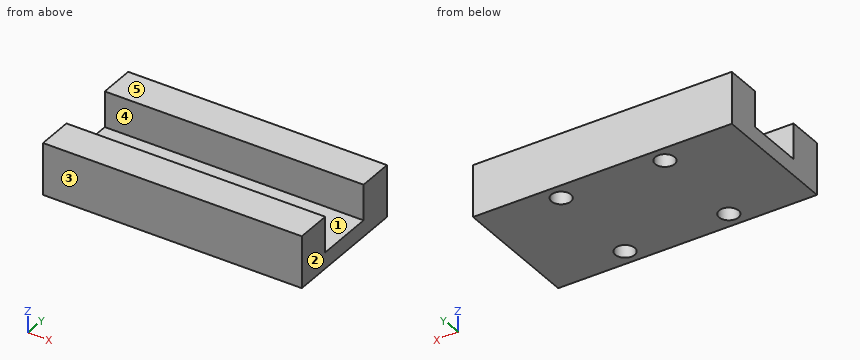
```python
from build123d import *

# Parameters (mm, degrees)
SKETCH_1_W          = 39.9
SKETCH_1_H          = 20
EXTRUDE_1_DEPTH     = 8
SKETCH_2_R          = 1.5
CUT_EXTRUDE_1_DEPTH = 3
SKETCH_3_W          = 5.5
SKETCH_3_H          = 9
CUT_EXTRUDE_2_DEPTH = 46.343246465


with BuildPart() as part:
    # 草图1 → 凸台-拉伸1 (new body)
    with BuildSketch(Plane.XY):
        with Locations((-19.95, 10)):
            Rectangle(SKETCH_1_W, SKETCH_1_H)
    extrude(amount=EXTRUDE_1_DEPTH)

    # 草图2 → 切除-拉伸1 (cut)
    with BuildSketch(Plane(origin=(0, 0, 0), x_dir=(-1, 0, 0), z_dir=(0, 0, -1))):
        with Locations((11.95, 17.5)):
            Circle(SKETCH_2_R)
        with Locations((27.95, 17.5)):
            Circle(SKETCH_2_R)
        with Locations(Location((27.95, 2.5, 0), (0, 0, 180))):
            Circle(SKETCH_2_R)
        with Locations(Location((11.95, 2.5, 0), (0, 0, 180))):
            Circle(SKETCH_2_R)
    extrude(amount=-CUT_EXTRUDE_1_DEPTH, mode=Mode.SUBTRACT)

    # 草图3 → 切除-拉伸2 (cut, through all)
    with BuildSketch(Plane(origin=(0, 0, 0), x_dir=(0, 0, -1), z_dir=(1, 0, 0))):
        with Locations((-5.25, 10)):
            Rectangle(SKETCH_3_W, SKETCH_3_H)
    extrude(amount=-CUT_EXTRUDE_2_DEPTH, mode=Mode.SUBTRACT)


solid = part.part
```
Check sheet for the modelled part. Datum: model origin and axes. Units: mm. Face numbers are marked on the shaded views. A direction names the side the tool comes from. Round coordinates to 2 decimals unless told otherwise and drop trailing zeros. Order: outer loops, then holes, each group sorted by start corner. A loop starts at its lowest first (then second) coordinate and runs counter-clockwise, first axis right, second up.
1) Go/stop test with flat-tipped pins: pin 1 Ø1.8 at (x, y) = (-11.95, 2.5) entering from -Z; pin 2 Ø4.5 at (x, y) = (-21.5, 10.5) entering from +Z. Record where each tip stops, or that it passes through.
2) Section check A-A (z = 4.5). Record the boundary of the cut face in (x, y), and give its area (3 significant figures).
3) Section check D-D (y = 1.5). Record the boundary of the cut face in (x, z), and give its area (3 significant figures).
4) Mould release check, pull along Y, two halves, no side actions. Record for the marked faces 1, 2 and 3: +Y half, -Y half, draft (parallel to the pull), parting line (faces both ways), or undercut.
5) Scan lines: line 1 (Y direction, x = -11.95, z = 2.1); line 2 (X direction, y = 2.5, z = 1.2); line 3 (Y direction, x = -20.5, z = 7.5). Record each from-to range of solid material in increasing order.
6) Section check C-C (x = -27.95). Record the boundary of the cut face in (y, z), and give its area (3 significant figures).
7) Section check B-B (z = 1.25). Record the boundary of the cut face in (x, y), and give its area (3 significant figures).
8) Tool access check on the marked faces 4 and 5. Record the directions out of +Z, -Z, +X, -X, +Y, -Y that give a thin tool (end or side, any length) a straight path to the whole face; none if there is none.
Result:
1. pin 1: stops at z = 3
1. pin 2: stops at z = 2.5
2. outline: (-39.9, 0) - (0, 0) - (0, 5.5) - (-39.9, 5.5) - close; (-39.9, 14.5) - (0, 14.5) - (0, 20) - (-39.9, 20) - close
2. area: 439 mm2
3. outline: (-39.9, 0) - (-29.07, 0) - (-29.07, 3) - (-26.83, 3) - (-26.83, 0) - (-13.07, 0) - (-13.07, 3) - (-10.83, 3) - (-10.83, 0) - (0, 0) - (0, 8) - (-39.9, 8) - close
3. area: 306 mm2
4. face 1: undercut
4. face 2: draft
4. face 3: -Y half
5. line 1: y = 0 to 1, 4 to 16, 19 to 20
5. line 2: x = -39.9 to -29.45, -26.45 to -13.45, -10.45 to 0
5. line 3: y = 0 to 5.5, 14.5 to 20
6. outline: (0, 0) - (1, 0) - (1, 3) - (4, 3) - (4, 0) - (16, 0) - (16, 3) - (19, 3) - (19, 0) - (20, 0) - (20, 8) - (14.5, 8) - (14.5, 2.5) - (5.5, 2.5) - (5.5, 8) - (0, 8) - close
6. area: 92.5 mm2
7. outline: (-39.9, 0) - (0, 0) - (0, 20) - (-39.9, 20) - close; hole circle Ø3 at (-27.95, 2.5); hole circle Ø3 at (-27.95, 17.5); hole circle Ø3 at (-11.95, 2.5); hole circle Ø3 at (-11.95, 17.5)
7. area: 770 mm2
8. face 4: +Z, +X, -X
8. face 5: +Z, +X, -X, +Y, -Y
